The model under review builds one solid part; all positions refer to its coordinate system, in mm. Round coordinates to 2 decimals unless told otherwise and drop trailing zeros. Write each loop counter-clockwise with the first axis right and the second up, starting at its lowest first coordinate (ties: lowest second). Pieces come first, ordered by that corner, then holes. Notation, with made-up numbers: (40.5, 52.5) -> (47.5, 52.5) arc R19 ccw to (47.5, 68.5) -> close; hole circle Ø4 at (-26, -3.5). An arc over 180 degrees is marked (long way). Return JSON: item names as keys, results as strings. Group by question number.
1. Take a section at C-C, the plane y = 16.5. Write out the cut boundary in (x, z), then the cut area to 3 significant figures.
2. Take a section at B-B, the plane z = 37. Write out the cut boundary in (x, y), then the cut area to 3 significant figures.
3. Mouldability with a two-part tool opening along Y and no side actions: class faces 1 (the flat face through (47, 5, 33)), 2 (the flat face through (0, 4.5, 21.3)), 3 (the flat face through (46.835, 27.185, 6.755)), 4 (the flat face through (47, 0, 30)) as pulls with the +Y half, pulls with the -Y half, needs draft (parallel to the pull), parting line crosses it, or undercut.
4. For line 1 along Y through (x, z) = (23.5, 54.5); line 2 along Z through (x, y) = (86, 17.5); line 3 along Z through (x, y) = (77, 33), list the stretches that pass through material, from the lowest coordinate up. Write a range as from..to.
5. Take a section at A-A, the plane x = 34. Write out the cut boundary in (y, z).
6. Clearance check with flat-ended pins moving along their axes: P1, Ø1.5, axis at x = 64.5, y = 9.5, coming from the -Z side; P2, Ø1.5, axis at x = 17, y = 19, coming from the +Z side; P3, Ø16, axis at x = 40.5, z = 29.5, coming from the +Y side. State where each tip first meets the part, or that it passes through.
from build123d import *

# Parameters (mm, degrees)
SKETCH1_W           = 95
SKETCH1_H           = 60
BOSS_EXTRUDE1_DEPTH = 5
BOSS_EXTRUDE3_DEPTH = 95


with BuildPart() as part:
    # Sketch1 → Boss-Extrude1 (new body)
    with BuildSketch(Plane(origin=(0, 0, 0), x_dir=(1, 0, 0), z_dir=(0, 1, 0))):
        with Locations((47.5, -30)):
            Rectangle(SKETCH1_W, SKETCH1_H)
    extrude(amount=BOSS_EXTRUDE1_DEPTH)

    # Sketch6 → Boss-Extrude3 (add)
    with BuildSketch(Plane.ZY):
        Polygon((0, 0), (12.424467848, 50), (17.424467848, 50), (16.182021063, 45), (5, 0), align=None)
    extrude(amount=-BOSS_EXTRUDE3_DEPTH)


solid = part.part
Output:
{
 "1": {"outline": "(0, 4.1) -> (95, 4.1) -> (95, 9.1) -> (0, 9.1) -> close", "area": "475 mm^2"},
 "2": {"outline": "(0, 0) -> (95, 0) -> (95, 5) -> (0, 5) -> close", "area": "475 mm^2"},
 "3": {"face 1": "undercut", "face 2": "needs draft", "face 3": "pulls with the +Y half", "face 4": "pulls with the -Y half"},
 "4": {"line 1": "y = 0..5", "line 2": "z = 4.35..9.35", "line 3": "z = 8.2..13.2"},
 "5": {"outline": "(0, 0) -> (5, 0) -> (5, 1.24) -> (50, 12.42) -> (50, 17.42) -> (5, 6.24) -> (5, 60) -> (0, 60) -> close"},
 "6": {"P1": "stops at z = 2.17", "P2": "stops at z = 9.91", "P3": "stops at y = 5"}
}
